Answer from the drawing. Dimensions are ordinates in mm from the lowest x, y and z of the part. A direction names the side the tool comes from. Give positions to 0.01 mm unless a question says otherwise; leave off trailing zeros. Write each loop counter-clockwise with the first axis right and the second up, starting at its lowest first coordinate (ties: lowest second). Pieces come first, ordered by that corner, then holes.
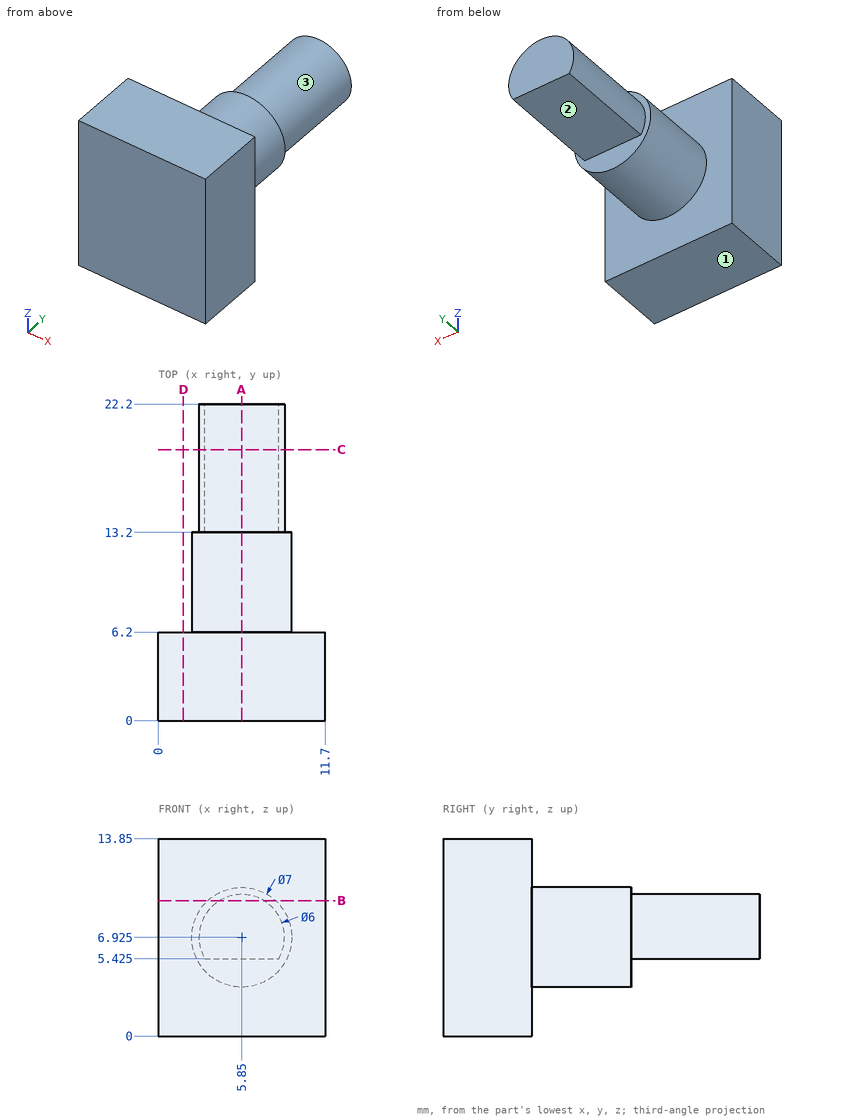
Item 1: A cutting plane is placed at C-C, the plane y = 19. Give the vertices of the cut face in (x, z) (3 decimals), plus the area to 3 significant figures.
Conclusion:
outline: (3.252, 5.425) - (8.448, 5.425) arc R3 ccw (long way) to start
area: 22.7 mm2
Item 2: Which of the six approach directions +Z, -Z, +X, -X, +Y, -Y give full straight-line access (tool end or side, diameter ignored) to the marked faces 1, 2 and 3?
Conclusion:
face 1: -Z, +X, -X, +Y, -Y
face 2: -Z, +X, -X, +Y
face 3: +Y
Item 3: A cutting plane is placed at A-A, the plane x = 5.85. Give the vertices of the cut face in (y, z) (3 decimals).
Conclusion:
outline: (0, 0) - (6.2, 0) - (6.2, 3.425) - (13.2, 3.425) - (13.2, 5.425) - (22.2, 5.425) - (22.2, 9.925) - (13.2, 9.925) - (13.2, 10.425) - (6.2, 10.425) - (6.2, 13.85) - (0, 13.85) - close
Item 4: A cutting plane is placed at D-D, the plane x = 1.75. Give the vertices of the cut face in (y, z).
Conclusion:
outline: (0, 0) - (6.2, 0) - (6.2, 13.85) - (0, 13.85) - close
Item 5: A cutting plane is placed at B-B, the plane z = 9.5. Give the vertices of the cut face in (x, y), plus the area to 3 significant figures.
Conclusion:
outline: (0, 0) - (11.7, 0) - (11.7, 6.2) - (8.22, 6.2) - (8.22, 13.2) - (7.39, 13.2) - (7.39, 22.2) - (4.31, 22.2) - (4.31, 13.2) - (3.48, 13.2) - (3.48, 6.2) - (0, 6.2) - close
area: 133 mm2
Item 6: Consider probe 1 along Y at (x, z) = (7, 13); probe 2 along Y at (x, z) = (2.5, 6.5); probe 3 along X at (y, z) = (14, 8.75). Determine where each line is inside the solid, lowest interval first.
Conclusion:
probe 1: y = 0 to 6.2
probe 2: y = 0 to 13.2
probe 3: x = 3.47 to 8.23
Item 7: Each of these flat-tipped pins is pushed along its axis until it touches: P1, Ø3, axis at y = 16, z = 7.5, coming from the -X side; P2, Ø2, axis at x = 3, y = 19, coming from the +Z side; P3, Ø4, axis at x = 6, y = 17.5, coming from the -Z side (3 decimals). Where does it stop, or does it pass through?
Conclusion:
P1: stops at x = 2.85
P2: stops at z = 9.29
P3: stops at z = 5.425
